Verification items for the finished model (mm, model axes). A direction names the side the tool comes from. Give positions to 0.01 mm unless a question says otherwise; leave off trailing zeros. Loops run counter-clockwise (first coordinate to the right, second up) from the corner with the lowest first, then second, coordinate; pieces in that order, holes last. Notation, with made-up numbers: M -27.75,-25.75 L -20.75,-25.75 A29 ccw -20.75,-3.75 Z; hole C -11.5,76.25 d2. An arc over 180 degrees is marked long. Write each question's results on one line, items separated by ' | '. Start each with the question number.
```python
from build123d import *

# Parameters (mm, degrees)
ESQUISSE1_R        = 85
BOSS_EXTRU_1_DEPTH = 150
ESQUISSE2_W        = 180
ESQUISSE2_H        = 180
BOSS_EXTRU_2_DEPTH = 20
CONG_1_R           = 5
CONG_2_R           = 5
CONG_3_R           = 5
CONG_4_R           = 5
CONG_5_R           = 5


with BuildPart() as part:
    # Esquisse1 → Boss.-Extru.1 (new body)
    with BuildSketch(Plane.XY):
        Circle(ESQUISSE1_R)
    extrude(amount=BOSS_EXTRU_1_DEPTH)

    # Esquisse2 → Boss.-Extru.2 (add)
    with BuildSketch(Plane.XY.offset(150)):
        Rectangle(ESQUISSE2_W, ESQUISSE2_H)
    extrude(amount=BOSS_EXTRU_2_DEPTH)

    # Congé1
    cong_1_edges = [part.edges().sort_by_distance(p)[0] for p in [
        (-85, 0, 150),
    ]]
    fillet(cong_1_edges, radius=CONG_1_R - 0.0001)  # a hair under: the kernel refuses the full size

    # Congé2
    cong_2_edges = [part.edges().sort_by_distance(p)[0] for p in [
        (-90, 90, 160),
    ]]
    fillet(cong_2_edges, radius=CONG_2_R)

    # Congé3
    cong_3_edges = [part.edges().sort_by_distance(p)[0] for p in [
        (-90, -90, 160),
    ]]
    fillet(cong_3_edges, radius=CONG_3_R)

    # Congé4
    cong_4_edges = [part.edges().sort_by_distance(p)[0] for p in [
        (90, 90, 160),
    ]]
    fillet(cong_4_edges, radius=CONG_4_R)

    # Congé5
    cong_5_edges = [part.edges().sort_by_distance(p)[0] for p in [
        (90, -90, 160),
    ]]
    fillet(cong_5_edges, radius=CONG_5_R)


solid = part.part
```
1. Section check C-C, the plane z = 92. Record the boundary of the cut face in (x, y).
2. Depth check by flat-ended pin: pin 1 Ø8 at (x, z) = (33.5, 116) entering from -Y; pin 2 Ø2 at (y, z) = (-51, 91) entering from -X; pin 3 Ø3 at (x, z) = (-66, 77.5) entering from -Y. Enter the tip coordinate at first touch or a pass-through.
3. Thickness scan on probe 1 along Z at (x, y) = (-56, 74); probe 2 along Y at (x, z) = (-45, 20.5); probe 3 along Y at (x, z) = (27, 117). Record the ranges inside material, lowest first.
4. Set-up check for faces 1 (the face through (-67.453, -51.721, 71.485)), 2 (the face through (-89, -88, 160)): record each of +Z, -Z, +X, -X, +Y, -Y from which the full face is reachable in a straight line by a thin tool's end or side.
Filled sheet:
1) outline: C 0,0 d170
2) pin 1: y = -79.72 | pin 2: x = -68.74 | pin 3: y = -55.36
3) probe 1: 150 to 170 | probe 2: -72.11 to 72.11 | probe 3: -80.6 to 80.6
4) face 1: -Z | face 2: +Z, -Z, -X, -Y
